Check sheet for the drawn part. Datum: minimum x, y, z corner. Units: mm. A direction names the side the tool comes from. Give positions to 0.01 mm unless a question says otherwise; leave off trailing zeros. Write each loop counter-clockwise with the first axis right and the second up, starting at its lowest first coordinate (ties: lowest second). Pieces come first, ordered by that corner, then holes. Notation, with made-up numbers: M 32,31 L 49,31 A19 ccw 49,51 Z; hole C 45,7.5 d7. An arc over 180 degrees is marked long. Use CSV: the item, a comma, the result in double quotes. Start each with the question number.
1. Depth check by flat-ended pin: P1, Ø1.5, axis at y = 13.5, z = 5.5, coming from the -X side. Enter the tip coordinate at first touch or a pass-through.
2. Mould release check, pull along Z, two halves, no side actions. Record for the marked faces 1, 2 and 3: +Z half, -Z half, draft (parallel to the pull), parting line (faces both ways), or undercut.
3. Scan lines: line 1 (Z direction, x = 3.5, y = 16.25); line 2 (Y direction, x = 4.5, z = 3); line 3 (Z direction, x = 2, y = 11.5) (1 decimal). Record each from-to range of solid material in increasing order.
4. Cross-section at A-A, the plane z = 3.5. Enter the section's corners in (x, y), and give its area (3 significant figures).
5. Cross-section at B-B, the plane y = 2.75. Enter the section's corners in (x, z), and give its area (3 significant figures).
6. Cross-section at D-D, the plane y = 16.75. Enter the section's corners in (x, z), and give its area (3 significant figures).
7. Cross-section at C-C, the plane x = 3.5. Enter the section's corners in (y, z).
8. Access from +Z, -Z, +X, -X, +Y, -Y to the whole of each face (thin tool, end or side, straight path). Record for the marked faces 4 and 5.
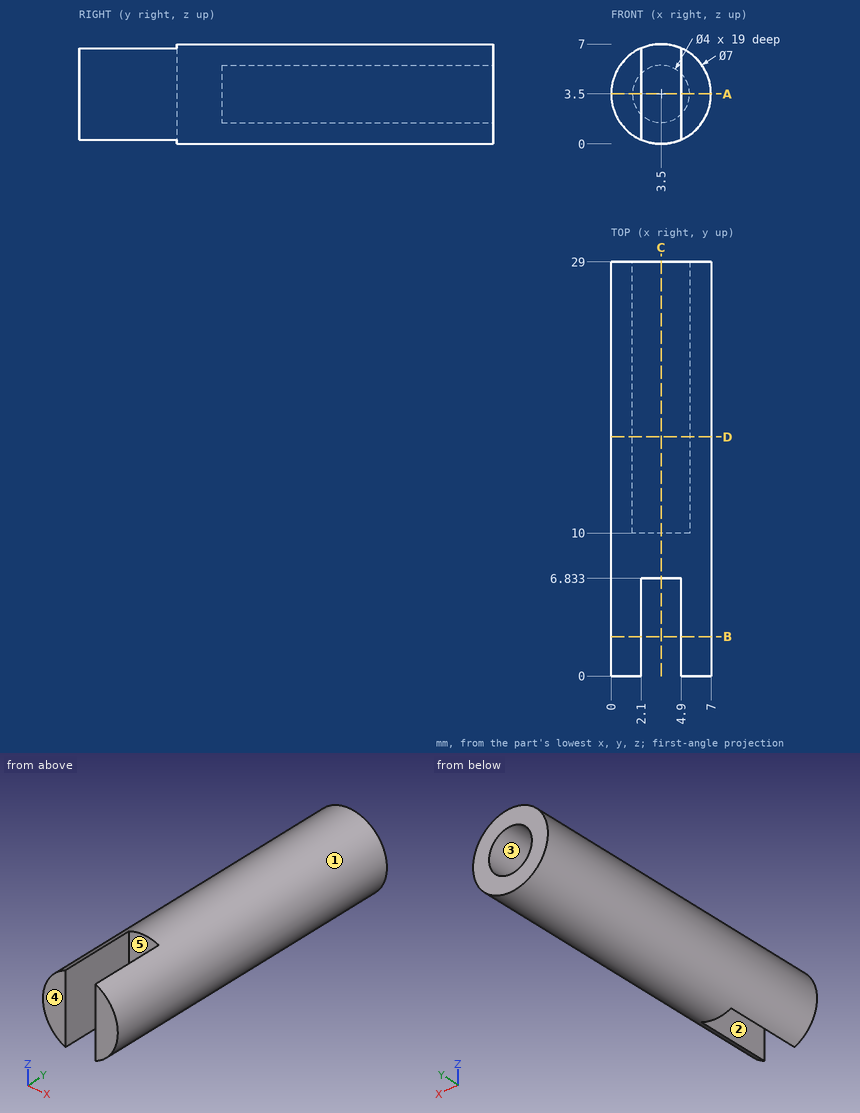
Worked answers:
1,P1,"stops at x = 0.23"
2,face 1,"parting line"
2,face 2,"draft"
2,face 3,"undercut"
3,line 1,"z = 0 to 1.5, 5.5 to 7"
3,line 2,"y = 6.83 to 10"
3,line 3,"z = 0.3 to 2.2, 4.8 to 6.7"
4,outline,"M 0,0 L 2.1,0 L 2.1,6.83 L 4.9,6.83 L 4.9,0 L 7,0 L 7,29 L 5.5,29 L 5.5,10 L 1.5,10 L 1.5,29 L 0,29 Z"
4,area,"108 mm^2"
5,outline,"M 2.1,0.29 L 2.1,6.71 A3.5 ccw Z; M 4.9,0.29 A3.5 ccw 4.9,6.71 Z"
5,area,"19.4 mm^2"
6,outline,"C 3.5,3.5 d7; hole C 3.5,3.5 d4"
6,area,"25.9 mm^2"
7,outline,"M 6.83,0 L 29,0 L 29,1.5 L 10,1.5 L 10,5.5 L 29,5.5 L 29,7 L 6.83,7 Z"
8,face 4,"+Z, -Z, +X, -X, -Y"
8,face 5,"+Z, -Z, -Y"
